Verification items for the finished model (mm, model axes). Face numbers are marked on the shaded views. A direction names the side the tool comes from. Round coordinates to 2 decimals unless told otherwise and drop trailing zeros. Order: outer loops, then holes, each group sorted by start corner. A loop starts at its lowest first (then second) coordinate and runs counter-clockwise, first axis right, second up. Notation, with made-up numbers: (73, 31.5) -> (110, 31.5) arc R18 cw to (110, 43.5) -> close; hole circle Ø4 at (80.5, 40). An arc over 180 degrees is marked (long way). Answer in a Markdown table with one row per item. Add a question column.
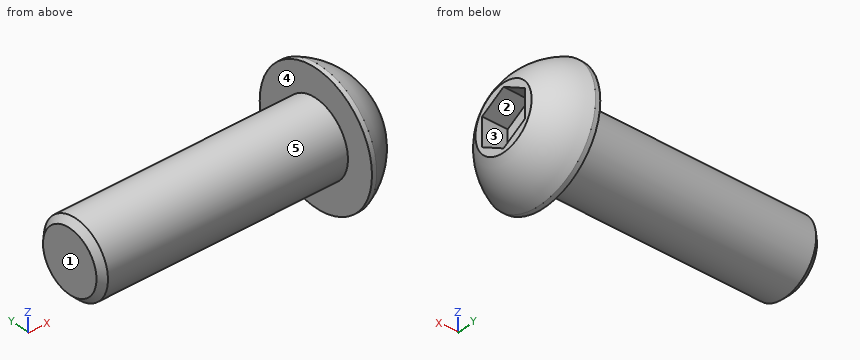
```python
from build123d import *

# Parameters (mm, degrees)
CUT_EXTRUDE1_DEPTH = 2.08
CHAMFER1_SIZE      = 0.5


with BuildPart() as part:
    # Sketch1 → Revolve1 (revolve)
    with BuildSketch(Plane.XY):
        with BuildLine():
            Line((0, 0), (0, 2.625))
            ThreePointArc((0, 2.625), (-1.224500646, 4.199464996), (-2.92, 5.25))
            Line((-2.92, 5.25), (-3.3, 5.25))
            Line((-3.3, 5.25), (-3.3, 3))
            Line((-3.3, 3), (-23.3, 3))
            Line((-23.3, 3), (-23.3, 0))
            Line((-23.3, 0), (0, 0))
        make_face()
    revolve(axis=Axis((0, 0, 0), (-1, 0, 0)))

    # Sketch2 → Cut-Extrude1 (cut)
    with BuildSketch(Plane(origin=(0, 0, 0), x_dir=(0, 0, -1), z_dir=(1, 0, 0))):
        Polygon((2.309401077, 0), (1.154700538, 2), (-1.154700538, 2), (-2.309401077, 0), (-1.154700538, -2), (1.154700538, -2), align=None)
    extrude(amount=-CUT_EXTRUDE1_DEPTH, mode=Mode.SUBTRACT)

    # Chamfer1
    chamfer1_edges = [part.edges().sort_by_distance(p)[0] for p in [
        (-23.3, -3, 0),
    ]]
    chamfer(chamfer1_edges, length=CHAMFER1_SIZE)


solid = part.part
```
1) Cross-section at B-B, the plane x = -15.75. Record the boundary of the cut face in (y, z), and give its area (3 significant figures).
2) Depth check by flat-ended pin: P1, Ø1.5, axis at x = -17, y = 4, coming from the +Z side; P2, Ø0.6, axis at x = -1, z = 0, coming from the +Y side; P3, Ø1, axis at x = -11.5, y = 0, coming from the +Z side; P4, Ø1, axis at x = -7, y = 0.5, coming from the -Z side. Enter the tip coordinate at first touch or a pass-through.
3) Tool access check on the marked faces 1 and 2. Record the directions out of +Z, -Z, +X, -X, +Y, -Y that give a thin tool (end or side, any length) a straight path to the whole face; none if there is none.
4) Draft check along Y on the marked faces 3, 4 and 5. Enter one of: +Y half, -Y half, draft (parallel to the pull), parting line (faces both ways), or undercut.
5) Cross-section at A-A, the plane z = 0. Record the boundary of the cut face in (x, y) (3 decimals).
6) Thickness scan on L1, parallel to X at y = 1.25, z = 1; L2, parallel to Z at x = -7, y = 0; L3, parallel to Z at x = -14.5, y = -2. Record the ranges inside material, lowest first. Write a range as [from, to].
7) Cross-section at C-C, the plane z = -4. Record the boundary of the cut face in (x, y).
Results below:
| question | item | result |
|---|---|---|
| 1 | outline | circle Ø6 at (0, 0) |
| 1 | area | 28.3 mm² |
| 2 | P1 | through |
| 2 | P2 | y = 4.27 |
| 2 | P3 | z = 3 |
| 2 | P4 | z = -3 |
| 3 | face 1 | +Z, -Z, -X, +Y, -Y |
| 3 | face 2 | +X |
| 4 | face 3 | undercut |
| 4 | face 4 | draft |
| 4 | face 5 | parting line |
| 5 | outline | (-23.3, -2.5) -> (-22.8, -3) -> (-3.3, -3) -> (-3.3, -5.25) -> (-2.92, -5.25) arc R5.647 ccw to (0, -2.625) -> (0, -2) -> (-2.08, -2) -> (-2.08, 2) -> (0, 2) -> (0, 2.625) arc R5.647 ccw to (-2.92, 5.25) -> (-3.3, 5.25) -> (-3.3, 3) -> (-22.8, 3) -> (-23.3, 2.5) -> close |
| 6 | L1 | [-23.3, -2.08] |
| 6 | L2 | [-3, 3] |
| 6 | L3 | [-2.24, 2.24] |
| 7 | outline | (-3.3, -3.4) -> (-2.92, -3.4) arc R3.99 ccw to (-2.92, 3.4) -> (-3.3, 3.4) -> close |
